```python
from build123d import *

# Parameters (mm, degrees)
F2_R     = 2.5
F0_DEPTH = 8.6
F3_DEPTH = 1.1
F4_R     = 2


with BuildPart() as f0:
    # F2 (on Top) → F0 (new body)
    with BuildSketch(Plane.XY):
        Circle(F2_R)
    extrude(amount=F0_DEPTH)

    # F1 (on Top) → F3 (join)
    with BuildSketch(Plane.XY):
        with BuildLine():
            Line((2.5, -1.469694), (2.5, 1.469694))
            ThreePointArc((2.5, 1.469694), (-2.9, 0), (2.5, -1.469694))
        make_face()
    extrude(amount=F3_DEPTH)

    # F4
    f4_edges = [f0.edges().sort_by_distance(p)[0] for p in [
        (-2.5, 0, 8.6),
    ]]
    fillet(f4_edges, radius=F4_R)


solid = f0.part
```
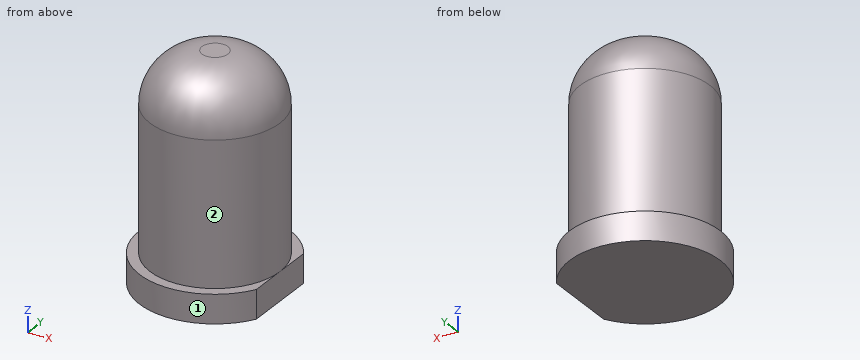
Work out the finished part from the listing and answer in its coordinate system (mm). Face numbers are marked on the shaded views. A direction names the side the tool comes from. Round coordinates to 2 decimals unless told otherwise and drop trailing zeros. Loops run counter-clockwise (first coordinate to the right, second up) from the corner with the lowest first, then second, coordinate; pieces in that order, holes last.
(1) Find the intervals of material crossed by L1, parallel to Z at x = 1.55, y = 2.15; L2, parallel to Z at x = -0.7, y = -1.4; L3, parallel to Y at x = -2.25, z = 2.5, in increasing order.
Computed values:
L1: z = 0 to 1.1
L2: z = 0 to 8.29
L3: y = -1.09 to 1.09
(2) The part is cut by section A-A, the plane z = 3.75. Give the vertices of the cut face in (x, y).
Computed values:
outline: circle Ø5 at (0, 0)
(3) Each of these flat-tipped pins is pushed along its axis until it touches: P1, Ø1.5, axis at x = -1, z = 2.5, coming from the +Y side; P2, Ø1, axis at y = 1, z = 4.5, coming from the +X side; P3, Ø2, axis at y = -2.5, z = 4, coming from the -X side. Where does it stop, or does it pass through?
Computed values:
P1: stops at y = 2.49
P2: stops at x = 2.45
P3: stops at x = -2
(4) For the marked faces 1 and 2, determine the directions among +Z, -Z, +X, -X, +Y, -Y from which every point of the face is accessible in a straight line to the end or side of a thin tool.
Computed values:
face 1: +Z, -Z
face 2: +Z
